```python
from build123d import *

# Parameters (mm, degrees)
F0_W     = 74
F0_H     = 16
F1_DEPTH = 6
F2_R     = 5
F3_DEPTH = 1.2
F4_SIZE  = 2


# Not quite as in the source:
# - a feature of the source that left no trace in its solid (it failed there, or was rolled back) is left out


with BuildPart() as f1:
    # F0 (on Top) → F1 (new body)
    with BuildSketch(Plane.XY):
        Rectangle(F0_W, F0_H)
    extrude(amount=F1_DEPTH)

    # F2 (on face) → F3 (cut)
    with BuildSketch(Plane.XY.offset(6)):
        with Locations((-24, 0)):
            Circle(F2_R)
        Circle(F2_R)
        with Locations((24, 0)):
            Circle(F2_R)
    extrude(amount=-F3_DEPTH, mode=Mode.SUBTRACT)

    # F4
    f4_edges = [f1.edges().sort_by_distance(p)[0] for p in [
        (-37, 8, 3),
        (-37, -8, 3),
        (37, -8, 3),
        (37, 8, 3),
        (-37, 0, 6),
        (37, 0, 6),
    ]]
    chamfer(f4_edges, length=F4_SIZE)


solid = f1.part
```
Geometry: final body of the model. Coordinates: model frame, mm. A direction names the side the tool comes from. Round coordinates to 2 decimals unless told otherwise and drop trailing zeros. Write each loop counter-clockwise with the first axis right and the second up, starting at its lowest first coordinate (ties: lowest second). Pieces come first, ordered by that corner, then holes.
Item 1: Mould query, pull axis X, two halves, no side actions, for faces 1 (the face through (-36, -7, 2)), 2 (the face through (36, -7, 2)), 3 (the face through (19, 0, 5)). Classes: +X half, -X half, draft (parallel to the pull), parting line (faces both ways), or undercut.
Item 2: Material intervals for L1, parallel to X at y = -3.75, z = 5; L2, parallel to X at y = -4.5, z = 5.4; L3, parallel to Y at x = -24, z = 5.6, sorted ascending.
Item 3: Set-up query: faces 4 (the face through (36, 7, 2)), 5 (the face through (-1.08, -4.88, 5.41)). Return all of +Z, -Z, +X, -X, +Y, -Y with unobstructed straight access to the full face (end or side cutting, diameter ignored); none if empty.
Item 4: Section query A-A (x = 0). Return loops of the section in (y, z).
Item 5: Section query C-C (y = 0). Return loops of the section in (x, z), plus the area to 3 significant figures.
Item 6: Section query B-B (y = 3). Return loops of the section in (x, z), plus the area to 3 significant figures.
Item 7: Section query D-D (y = 7). Return loops of the section in (x, z).
Completed:
1. face 1: -X half
1. face 2: +X half
1. face 3: undercut
2. L1: x = -36 to -27.31, -20.69 to -3.31, 3.31 to 20.69, 27.31 to 36
2. L2: x = -35.6 to -26.18, -21.82 to -2.18, 2.18 to 21.82, 26.18 to 35.6
2. L3: y = -8 to -5, 5 to 8
3. face 4: +Z, -Z, +X, +Y
3. face 5: +Z
4. outline: (-8, 0) - (8, 0) - (8, 6) - (5, 6) - (5, 4.8) - (-5, 4.8) - (-5, 6) - (-8, 6) - close
5. outline: (-37, 0) - (37, 0) - (37, 4) - (35, 6) - (29, 6) - (29, 4.8) - (19, 4.8) - (19, 6) - (5, 6) - (5, 4.8) - (-5, 4.8) - (-5, 6) - (-19, 6) - (-19, 4.8) - (-29, 4.8) - (-29, 6) - (-35, 6) - (-37, 4) - close
5. area: 404 mm2
6. outline: (-37, 0) - (37, 0) - (37, 4) - (35, 6) - (28, 6) - (28, 4.8) - (20, 4.8) - (20, 6) - (4, 6) - (4, 4.8) - (-4, 4.8) - (-4, 6) - (-20, 6) - (-20, 4.8) - (-28, 4.8) - (-28, 6) - (-35, 6) - (-37, 4) - close
6. area: 411 mm2
7. outline: (-36, 0) - (36, 0) - (36, 5) - (35, 6) - (-35, 6) - (-36, 5) - close
